Here's how the part is built. I have some questions about the finished solid (model axes, mm). Face numbers are marked on the shaded views. A direction names the side the tool comes from. Round coordinates to 2 decimals unless told otherwise and drop trailing zeros. Order: outer loops, then holes, each group sorted by start corner. A loop starts at its lowest first (then second) coordinate and runs counter-clockwise, first axis right, second up. Notation, with made-up numbers: (-19, 30.5) -> (16, 30.5) arc R16 ccw to (16, 58.5) -> close; hole circle Ø1 at (-13.75, 63.5). An arc over 180 degrees is marked (long way). One line per item, written item: value.
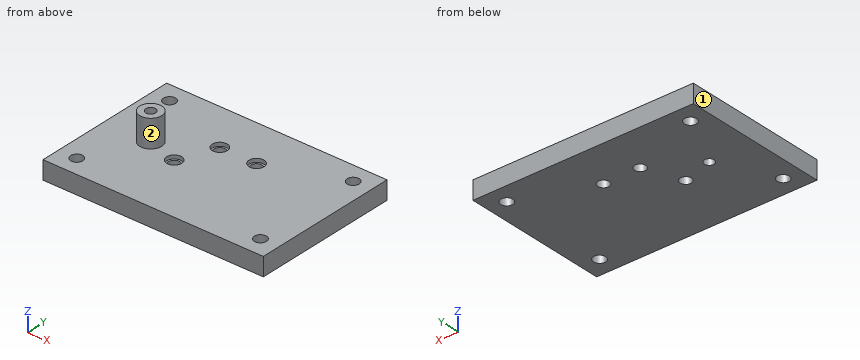
```python
from build123d import *

# Parameters (mm, degrees)
SKETCH2_W                          = 120
SKETCH2_H                          = 80
BASE_PLATE_DEPTH                   = 10
PIVOT_PEDESTAL_START               = 10
SKETCH3_R                          = 6
PIVOT_PEDESTAL_DEPTH               = 15
SKETCH4_R                          = 2.7
PIVOT_CLEARANCE_DEPTH              = 25
SKETCH5_R                          = 3.1
LOCATOR_CLEARANCE_DEPTH            = 10
SKETCH6_R                          = 3.1
CUT_EXTRUDE3_DEPTH                 = 10
SKETCH7_R                          = 3.1
SIDE_LOCATOR_CLEARANCE_DEPTH       = 10
LOCATOR_SHOULDER_COUNTERBORE_START = 8
SKETCH8_R                          = 4.1
LOCATOR_SHOULDER_COUNTERBORE_DEPTH = 2
CUT_EXTRUDE6_START                 = 8
SKETCH9_R                          = 4.1
CUT_EXTRUDE6_DEPTH                 = 2
SIDE_SHOULDER_COUNTERBORE_START    = 8
SKETCH10_R                         = 4.1
SIDE_SHOULDER_COUNTERBORE_DEPTH    = 2
SKETCH11_R                         = 3.3
BENCH_MOUNT_M6_CLEARANCE_DEPTH     = 10
SKETCH12_R                         = 3.3
CUT_EXTRUDE9_DEPTH                 = 10
SKETCH13_R                         = 3.3
CUT_EXTRUDE10_DEPTH                = 10
SKETCH14_R                         = 3.3
CUT_EXTRUDE11_DEPTH                = 10


with BuildPart() as part:
    # Sketch2 → Base_plate (new body)
    with BuildSketch(Plane.XY):
        Rectangle(SKETCH2_W, SKETCH2_H)
    extrude(amount=BASE_PLATE_DEPTH)

    # Sketch3 → Pivot_pedestal (add)
    with BuildSketch(Plane.XY.offset(PIVOT_PEDESTAL_START)):
        with Locations(Location((-35, 0, 0), (0, 0, 180))):
            Circle(SKETCH3_R)
    extrude(amount=PIVOT_PEDESTAL_DEPTH)

    # Sketch4 → Pivot_clearance (cut)
    with BuildSketch(Plane.XY):
        with Locations((-35, 0)):
            Circle(SKETCH4_R)
    extrude(amount=PIVOT_CLEARANCE_DEPTH, mode=Mode.SUBTRACT)

    # Sketch5 → Locator_clearance (cut)
    with BuildSketch(Plane.XY):
        with Locations((-10, 15)):
            Circle(SKETCH5_R)
    extrude(amount=LOCATOR_CLEARANCE_DEPTH, mode=Mode.SUBTRACT)

    # Sketch6 → Cut-Extrude3 (cut)
    with BuildSketch(Plane.XY):
        with Locations((10, 15)):
            Circle(SKETCH6_R)
    extrude(amount=CUT_EXTRUDE3_DEPTH, mode=Mode.SUBTRACT)

    # Sketch7 → Side_locator_clearance (cut)
    with BuildSketch(Plane.XY):
        with Locations((-18, -5)):
            Circle(SKETCH7_R)
    extrude(amount=SIDE_LOCATOR_CLEARANCE_DEPTH, mode=Mode.SUBTRACT)

    # Sketch8 → Locator_shoulder_counterbore (cut)
    with BuildSketch(Plane.XY.offset(LOCATOR_SHOULDER_COUNTERBORE_START)):
        with Locations((-10, 15)):
            Circle(SKETCH8_R)
    extrude(amount=LOCATOR_SHOULDER_COUNTERBORE_DEPTH, mode=Mode.SUBTRACT)

    # Sketch9 → Cut-Extrude6 (cut)
    with BuildSketch(Plane.XY.offset(CUT_EXTRUDE6_START)):
        with Locations((10, 15)):
            Circle(SKETCH9_R)
    extrude(amount=CUT_EXTRUDE6_DEPTH, mode=Mode.SUBTRACT)

    # Sketch10 → Side_shoulder_counterbore (cut)
    with BuildSketch(Plane.XY.offset(SIDE_SHOULDER_COUNTERBORE_START)):
        with Locations((-18, -5)):
            Circle(SKETCH10_R)
    extrude(amount=SIDE_SHOULDER_COUNTERBORE_DEPTH, mode=Mode.SUBTRACT)

    # Sketch11 → Bench_mount_M6_clearance (cut)
    with BuildSketch(Plane.XY):
        with Locations((-50, -30)):
            Circle(SKETCH11_R)
    extrude(amount=BENCH_MOUNT_M6_CLEARANCE_DEPTH, mode=Mode.SUBTRACT)

    # Sketch12 → Cut-Extrude9 (cut)
    with BuildSketch(Plane.XY):
        with Locations((-50, 30)):
            Circle(SKETCH12_R)
    extrude(amount=CUT_EXTRUDE9_DEPTH, mode=Mode.SUBTRACT)

    # Sketch13 → Cut-Extrude10 (cut)
    with BuildSketch(Plane.XY):
        with Locations((50, -30)):
            Circle(SKETCH13_R)
    extrude(amount=CUT_EXTRUDE10_DEPTH, mode=Mode.SUBTRACT)

    # Sketch14 → Cut-Extrude11 (cut)
    with BuildSketch(Plane.XY):
        with Locations((50, 30)):
            Circle(SKETCH14_R)
    extrude(amount=CUT_EXTRUDE11_DEPTH, mode=Mode.SUBTRACT)


solid = part.part
```
Q1. I want a section at A-A on x = 50. Write out the boundary of the cut face in (y, z), then the cut area to 3 significant figures.
Answers:
outline: (-40, 0) -> (-33.3, 0) -> (-33.3, 10) -> (-40, 10) -> close; (-26.7, 0) -> (26.7, 0) -> (26.7, 10) -> (-26.7, 10) -> close; (33.3, 0) -> (40, 0) -> (40, 10) -> (33.3, 10) -> close
area: 668 mm2
Q2. For P1, Ø8, axis at x = -45, y = -7.5, coming from the +Z side; P2, Ø4, axis at x = -32.5, z = 19, coming from the -Y side; P3, Ø5, axis at y = 0, z = 15.5, coming from the +X side, each with a flat end and sliding along its axis, tell me the tip position at first contact or that it passes through.
Answers:
P1: z = 10
P2: y = -5.98
P3: x = -29
Q3. I want a section at B-B on y = 15. Write out the boundary of the cut face in (x, z).
Answers:
outline: (-60, 0) -> (-13.1, 0) -> (-13.1, 8) -> (-14.1, 8) -> (-14.1, 10) -> (-60, 10) -> close; (-6.9, 0) -> (6.9, 0) -> (6.9, 8) -> (5.9, 8) -> (5.9, 10) -> (-5.9, 10) -> (-5.9, 8) -> (-6.9, 8) -> close; (13.1, 0) -> (60, 0) -> (60, 10) -> (14.1, 10) -> (14.1, 8) -> (13.1, 8) -> close
Q4. I want a section at D-D on z = 21.5. Write out the boundary of the cut face in (x, y).
Answers:
outline: circle Ø12 at (-35, 0); hole circle Ø5.4 at (-35, 0)
Q5. Which directions (+Z, -Z, +X, -X, +Y, -Y) give clear straight access to the entire face, cutting with the end or side of a thin tool? Please do the marked faces 1 and 2.
Answers:
face 1: +Z, -Z, -X, +Y, -Y
face 2: +Z
Q6. I want a section at C-C on x = -17.5. Write out the boundary of the cut face in (y, z), then the cut area to 3 significant figures.
Answers:
outline: (-40, 0) -> (-8.06, 0) -> (-8.06, 8) -> (-9.07, 8) -> (-9.07, 10) -> (-40, 10) -> close; (-1.94, 0) -> (40, 0) -> (40, 10) -> (-0.93, 10) -> (-0.93, 8) -> (-1.94, 8) -> close
area: 735 mm2
Q7. I need wall thicknesses on line 1 along X through (y, z) = (15, 6.75); line 2 along Y through (x, z) = (-50, 7.75); line 3 along X through (y, z) = (13, 1.25). Which ranges of each line are inside material? Lowest first, please.
Answers:
line 1: -60 to -13.1, -6.9 to 6.9, 13.1 to 60
line 2: -40 to -33.3, -26.7 to 26.7, 33.3 to 40
line 3: -60 to -12.37, -7.63 to 7.63, 12.37 to 60
